Could you check a few things on this model? Use its own coordinates, in mm. A direction names the side the tool comes from. Give positions to 0.01 mm unless a question says otherwise; leave off trailing zeros. Loops run counter-clockwise (first coordinate to the right, second up) from the corner with the lowest first, then second, coordinate; pieces in that order, holes last. Notation, with made-up numbers: (-6.75, 24) -> (15.25, 24) arc R10 cw to (15.25, 31) -> close; hole circle Ø11 at (32, -32.5). An arc over 180 degrees is marked (long way). Write item = value, one per line. Start each with the question number.
1) I want a section at D-D (y = 16.25). List the corners of the cut face in (x, z) for me.
2) If we mould it in two halves opening along X, with no side actions, what happens to faces 4 (the face through (-13, 24, 0)), 5 (the face through (2.703, 11.923, -8.584))? For each: +X half, -X half, draft (parallel to the pull), parting line (faces both ways), or undercut.
3) I need wall thicknesses on probe 1 along X at (y, z) = (3.75, 0); probe 2 along Z at (x, y) = (5.5, 6.25); probe 3 along X at (y, z) = (3.5, -6.5). Which ranges of each line are inside material? Lowest first, please. Write a range as from..to.
4) On a 3-axis mill with a long thin cutter (end or side, diameter ignored), from which of +Z, -Z, +X, -X, +Y, -Y can I reach the whole of each face in a straight line? I mean faces 1 (the face through (-9, 17.5, 2)), 2 (the face through (9, 6.5, 2)), 3 (the face through (-13, 0, 0)). Say none if no direction works.
5) I want a section at C-C (y = 4). List the corners of the cut face in (x, z) for me, and give its area (3 significant figures).
6) I'm going to push flat-ended pins straight in: pin 1 Ø12 at (x, y) = (-15.5, 5.5) entering from +Z; pin 2 Ø3 at (y, z) = (19.5, 8) entering from -X; pin 3 Ø6.5 at (x, z) = (3, 4.5) entering from +Y; pin 4 Ø6 at (y, z) = (7.5, -28) entering from -X. Where does each tip first touch, or does it pass through?
from build123d import *

# Parameters (mm, degrees)
SKETCH1_R           = 42
BOSS_EXTRUDE1_DEPTH = 24
FILLET1_R           = 12
SKETCH2_R           = 11
CUT_EXTRUDE1_DEPTH  = 6.5
CUT_EXTRUDE2_START  = -6.5
SKETCH3_R           = 11
CUT_EXTRUDE2_DEPTH  = 6.5
SKETCH4_R           = 9
CUT_EXTRUDE3_DEPTH  = 62.921321113


with BuildPart() as part:
    # Sketch1 → Boss-Extrude1 (new body)
    with BuildSketch(Plane(origin=(0, 0, 0), x_dir=(1, 0, 0), z_dir=(0, 1, 0))):
        with Locations(Location((0, 0, 0), (0, 0, 270))):
            Circle(SKETCH1_R)
    extrude(amount=BOSS_EXTRUDE1_DEPTH)

    # Fillet1
    fillet1_edges = [part.edges().sort_by_distance(p)[0] for p in [
        (0, 0, -42),
        (0, 24, -42),
    ]]
    fillet(fillet1_edges, radius=FILLET1_R - 0.0001)  # a hair under: the kernel refuses the full size

    # Sketch2 → Cut-Extrude1 (cut)
    with BuildSketch(Plane(origin=(0, 24, 0), x_dir=(1, 0, 0), z_dir=(0, 1, 0))):
        with Locations(Location((0, 0, 0), (0, 0, 270))):
            Circle(SKETCH2_R)
    extrude(amount=-CUT_EXTRUDE1_DEPTH, mode=Mode.SUBTRACT)

    # Sketch3 → Cut-Extrude2 (cut)
    with BuildSketch(Plane.XZ.offset(CUT_EXTRUDE2_START)):
        with Locations(Location((0, 0, 0), (0, 0, 90))):
            Circle(SKETCH3_R)
    extrude(amount=CUT_EXTRUDE2_DEPTH, mode=Mode.SUBTRACT)

    # Sketch4 → Cut-Extrude3 (cut, through all)
    with BuildSketch(Plane.XZ.offset(-6.5)):
        with Locations(Location((0, 0, 0), (0, 0, 270))):
            Circle(SKETCH4_R)
    extrude(amount=-CUT_EXTRUDE3_DEPTH, mode=Mode.SUBTRACT)


solid = part.part
Answer list:
q1.outline = circle Ø82.44 at (0, 0); hole circle Ø18 at (0, 0)
q2.face_4 = draft
q2.face_5 = undercut
q3.probe_1 = -38.71..-11, 11..38.71
q3.probe_2 = -40.16..-9.53, 9.53..40.16
q3.probe_3 = -37.92..-8.87, 8.87..37.92
q4.face_1 = +Y
q4.face_2 = -Y
q4.face_3 = +Z, -Z, +X, -X, -Y
q5.outline = circle Ø77.89 at (0, 0); hole circle Ø22 at (0, 0)
q5.area = 4,380 mm^2
q6.pin_1 = 40.25
q6.pin_2 = -39.64
q6.pin_3 = through
q6.pin_4 = -32.98
